from build123d import *
from build123d.topology import SkipClean

# Parameters (mm, degrees)
BODY_DEPTH         = 5
SKETCH4_R          = 2.5
TOP_ELECTRIC_DEPTH = 1
SKETCH6_R          = 0.75
CABLE_DEPTH        = 7.5


with BuildPart() as part:
    # Sketch1 → Body (new body)
    with BuildSketch(Plane.XY.offset(125.3)):
        with BuildLine():
            Line((-20.05, 9), (-17.6, 12.720551034))
            Line((-17.6, 12.720551034), (-17.6, 32.8))
            ThreePointArc((-17.6, 32.8), (-12.445079349, 45.245079349), (0, 50.4))
            ThreePointArc((0, 50.4), (12.445079349, 45.245079349), (17.6, 32.8))
            Line((17.6, 32.8), (17.6, 12.720551034))
            Line((17.6, 12.720551034), (20.05, 9))
            Line((20.05, 9), (20.05, 0))
            Line((20.05, 0), (20.05, -11.4))
            Line((20.05, -11.4), (11.588549493, -18.5))
            Line((11.588549493, -18.5), (7.016550666, -18.5))
            Line((7.016550666, -18.5), (-7.016550666, -18.5))
            Line((-7.016550666, -18.5), (-11.588549493, -18.5))
            Line((-11.588549493, -18.5), (-20.05, -11.4))
            Line((-20.05, -11.4), (-20.05, 0))
            Line((-20.05, 0), (-20.05, 9))
        make_face()
    extrude(amount=BODY_DEPTH)

    # Sketch3 → Motor-Body (revolve)
    with SkipClean():  # keep this step's faces unmerged: merging them makes the solid invalid here
        with BuildSketch(Plane(origin=(0, 0, 0), x_dir=(0, 0, -1), z_dir=(1, 0, 0)), mode=Mode.PRIVATE) as motor_body_sk:
            with BuildLine():
                Line((-125.3, 32.8), (-40.4, 32.8))
                Line((-40.4, 32.8), (-40.4, 36.490598923))
                Line((-40.4, 36.490598923), (-44.4, 38.8))
                Line((-44.4, 38.8), (-44.4, 47.9))
                ThreePointArc((-44.4, 47.9), (-45.132233047, 49.667766953), (-46.9, 50.4))
                Line((-46.9, 50.4), (-125.3, 50.4))
                Line((-125.3, 50.4), (-125.3, 32.8))
            make_face()
        revolve(motor_body_sk.sketch.rotate(Axis((0, 32.8, 140.3), (0, 0, -1)), 90), axis=Axis((0, 32.8, 140.3), (0, 0, -1)))  # turned: the seam where the file's is

    # Sketch4 → Top-Electric (add)
    with SkipClean():  # keep this step's faces unmerged: merging them makes the solid invalid here
        with BuildSketch(Plane(origin=(0, 0, 44.4), x_dir=(-1, 0, 0), z_dir=(0, 0, -1))):
            with Locations(Location((9.84807753, 31.063518223, 0), (0, 0, 180))):  # turned: the seam where the file's is
                Circle(SKETCH4_R)
            with Locations(Location((5, 41.460254038, 0), (0, 0, 180))):  # turned: the seam where the file's is
                Circle(SKETCH4_R)
        extrude(amount=TOP_ELECTRIC_DEPTH)

    # Sketch6 → Cable (add)
    with SkipClean():  # keep this step's faces unmerged: merging them makes the solid invalid here
        with BuildSketch(Plane(origin=(0, 0, 43.4), x_dir=(-1, 0, 0), z_dir=(0, 0, -1))):
            with Locations((5, 41.460254038)):
                Circle(SKETCH6_R)
            with Locations((9.84807753, 31.063518223)):
                Circle(SKETCH6_R)
        extrude(amount=CABLE_DEPTH)


solid = part.part
Geometry: final body of the model. Coordinates: model frame, mm. A direction names the side the tool comes from. Coordinates: 2 decimals unless noted, no trailing zeros. Loops run counter-clockwise (first coordinate to the right, second up) from the corner with the lowest first, then second, coordinate; pieces in that order, holes last. Notation, with made-up numbers: (67.5, 22.25) - (121.5, 22.25) arc R23 cw to (121.5, 42.25) - close; hole circle Ø8 at (22.25, -14.75). An arc over 180 degrees is marked (long way). Put each result on its own line as item: value. Start each with the question number.
Q1. Pin query (flat end, axial travel): pin 1 Ø6 at (x, z) = (-4, 66) entering from -Y; pin 2 Ø1 at (y, z) = (42, 107) entering from +X; pin 3 Ø1.5 at (x, y) = (-10.5, 30.5) entering from -Z; pin 4 Ø1.5 at (y, z) = (25.5, 127.5) entering from +X. Return the tip coordinate at first contact, or that it passes through.
Q2. Cut plane A-A, the plane z = 52. Return loops of the section in (x, y).
Q3. Set-up query: faces 1 (the flat face through (0, 33, 40.4)), 2 (the flat face through (0, 39, 44.4)), 3 (the flat face through (-17.6, 23, 128)). Return all of +Z, -Z, +X, -X, +Y, -Y with unobstructed straight access to the full face (end or side cutting, diameter ignored); none if empty.
Q4. Cut plane B-B, the plane z = 42. Return loops of the section in (x, y), and give its area (3 significant figures).
Q5. Line query: line 1 (Z direction, x = -12.5, y = 41); line 2 (Z direction, x = -11.5, y = 1); line 3 (X direction, y = 33.5, z = 126). Output: solid intervals per line, ascending.
Filled sheet:
1. pin 1: y = 15.23
1. pin 2: x = 15.3
1. pin 3: z = 35.9
1. pin 4: x = 17.6
2. outline: circle Ø35.2 at (0, 32.8)
3. face 1: -Z, +X, +Y, -Y
3. face 2: -Z
3. face 3: +Z, -Z, -X, +Y
4. outline: circle Ø1.5 at (-9.85, 31.06); circle Ø1.5 at (-5, 41.46); circle Ø9.23 at (0, 32.8)
4. area: 70.4 mm²
5. line 1: 44.4 to 130.3
5. line 2: 125.3 to 130.3
5. line 3: -17.59 to 17.59
